Check sheet for the modelled part. Datum: model origin and axes. Units: mm. A direction names the side the tool comes from. Round coordinates to 2 decimals unless told otherwise and drop trailing zeros. Write each loop counter-clockwise with the first axis right and the second up, starting at its lowest first coordinate (ties: lowest second). Pieces come first, ordered by that corner, then holes.
from build123d import *

# Parameters (mm, degrees)
ESQUISSE2_W                 = 220
ESQUISSE2_H                 = 30
T_LE_DE_BASE_PLI_E1_DEPTH   = 4
PLI_START                   = -15
PLI_ESQUISS_1_DEPTH         = 30
PLI_ESQUISS_1_2_DEPTH       = 30
ESQUISSE9_R                 = 4.5
ESQUISSE9_R_2               = 1.25
BOSS_EXTRU_1_DEPTH          = 1.5
ENL_V_START                 = -4
ENL_V_MAT_EXTRU_1_OUTLINE_R = 1.25
ENL_V_MAT_EXTRU_1_DEPTH     = 4
BOSS_EXTRU_2_DEPTH          = 12
BOSS_EXTRU_2_DEPTH_BACK     = 58
ESQUISSE11_W                = 2.5
ESQUISSE11_H                = 30
BOSS_EXTRU_3_DEPTH          = 3
ESQUISSE13_R                = 2
ENL_V_MAT_EXTRU_2_DEPTH     = 1.5
ENL_V_MAT_EXTRU_3_REACH     = 127.256
ESQUISSE14_W                = 1
ESQUISSE14_H                = 17
ESQUISSE12_R                = 1.75
ENL_V_MAT_EXTRU_4_DEPTH     = 223.720608774
ESQUISSE12_7_R              = 5.25
ESQUISSE12_7_R_2            = 1.75
ENL_V_MAT_EXTRU_5_DEPTH     = 223.720608774
BOSS_EXTRU_4_START          = -15
BOSS_EXTRU_4_DEPTH          = 30


# Read off the part's stored shape, not the designer's step: Pli esquissé1, Enlèv. mat.-Extru.1, Boss.-Extru.4
# Sheet-metal steps are written as plain solids
with BuildPart() as part:
    # Esquisse2 → Tôle de base pliée1 (new body)
    with BuildSketch(Plane(origin=(0, 0, 0), x_dir=(1, 0, 0), z_dir=(0, 1, 0))):
        Rectangle(ESQUISSE2_W, ESQUISSE2_H)
    extrude(amount=-T_LE_DE_BASE_PLI_E1_DEPTH)

    # Pli esquissé1 outline → Pli esquissé1 (cut)
    with BuildSketch(Plane.XY.offset(PLI_START)):
        with BuildLine():
            Line((110, 0), (87.480931171, 0))
            Line((87.480931171, 0), (81.651859795, -3.365415928))
            ThreePointArc((81.651859795, -3.365415928), (80.509482084, -3.838604269), (79.283559795, -4))
            Line((79.283559795, -4), (110, -4))
            Line((110, -4), (110, 0))
        make_face()
    extrude(amount=PLI_ESQUISS_1_DEPTH, mode=Mode.SUBTRACT)

    # Pli esquiss_1 2 outline → Pli esquiss_1 2 (add)
    with BuildSketch(Plane.XY.offset(PLI_START)):
        with BuildLine():
            Line((87.480931171, 0), (107.012166491, 11.27636397))
            Line((107.012166491, 11.27636397), (105.012166491, 14.740465585))
            Line((105.012166491, 14.740465585), (79.651859795, 0.098685688))
            ThreePointArc((79.651859795, 0.098685688), (79.474205904, 0.025099036), (79.283559795, 0))
            Line((79.283559795, 0), (87.480931171, 0))
        make_face()
    extrude(amount=PLI_ESQUISS_1_2_DEPTH)

    # Esquisse9 → Boss.-Extru.1 (add)
    # profile 1 of 4: a face of its own
    with BuildSketch(Plane(origin=(19.870232793, -34.416252755, 0), x_dir=(0.8660254037844382, 0.5000000000000011, 0), z_dir=(-0.5000000000000011, 0.8660254037844382, 0))):
        with Locations(Location((80.313436681, 10.5, 0), (0, 0, 90))):
            Circle(ESQUISSE9_R)
        with Locations(Location((80.313436681, 10.5, 0), (0, 0, 180))):
            Circle(ESQUISSE9_R_2, mode=Mode.SUBTRACT)
    # profile 2 of 4: a face of its own
    with BuildSketch(Plane(origin=(19.870232793, -34.416252755, 0), x_dir=(0.8660254037844382, 0.5000000000000011, 0), z_dir=(-0.5000000000000011, 0.8660254037844382, 0))):
        with Locations((93.813436681, 10.5)):
            Circle(ESQUISSE9_R)
        with Locations(Location((93.813436681, 10.5, 0), (0, 0, 180))):
            Circle(ESQUISSE9_R_2, mode=Mode.SUBTRACT)
    # profile 3 of 4: a face of its own
    with BuildSketch(Plane(origin=(19.870232793, -34.416252755, 0), x_dir=(0.8660254037844382, 0.5000000000000011, 0), z_dir=(-0.5000000000000011, 0.8660254037844382, 0))):
        with Locations((93.813436681, -10.5)):
            Circle(ESQUISSE9_R)
        with Locations((93.813436681, -10.5)):
            Circle(ESQUISSE9_R_2, mode=Mode.SUBTRACT)
    # profile 4 of 4: a face of its own
    with BuildSketch(Plane(origin=(19.870232793, -34.416252755, 0), x_dir=(0.8660254037844382, 0.5000000000000011, 0), z_dir=(-0.5000000000000011, 0.8660254037844382, 0))):
        with Locations((80.313436681, -10.5)):
            Circle(ESQUISSE9_R)
        with Locations((80.313436681, -10.5)):
            Circle(ESQUISSE9_R_2, mode=Mode.SUBTRACT)
    extrude(amount=BOSS_EXTRU_1_DEPTH)

    # Enlèv. mat.-Extru.1 outline → Enlèv. mat.-Extru.1 (cut)
    with BuildSketch(Plane(origin=(19.870232793, -34.416252755, 0), x_dir=(0.8660254037844382, 0.5000000000000011, 0), z_dir=(-0.5000000000000011, 0.8660254037844382, 0)).offset(ENL_V_START)):
        with Locations((93.813436681, 10.5)):
            Circle(ENL_V_MAT_EXTRU_1_OUTLINE_R)
        with Locations((93.813436681, -10.5)):
            Circle(ENL_V_MAT_EXTRU_1_OUTLINE_R)
        with Locations((80.313436681, 10.5)):
            Circle(ENL_V_MAT_EXTRU_1_OUTLINE_R)
        with Locations((80.313436681, -10.5)):
            Circle(ENL_V_MAT_EXTRU_1_OUTLINE_R)
    extrude(amount=ENL_V_MAT_EXTRU_1_DEPTH, mode=Mode.SUBTRACT)

    # Esquisse11 → Boss.-Extru.2 (add, two sides: drawn at the far end of the back side and taken through both)
    with BuildSketch(Plane(origin=(0, 0, 0), x_dir=(1, 0, 0), z_dir=(0, 1, 0)).offset(-BOSS_EXTRU_2_DEPTH_BACK)):
        with Locations((-108.75, 0)):
            Rectangle(ESQUISSE11_W, ESQUISSE11_H)
    extrude(amount=BOSS_EXTRU_2_DEPTH + BOSS_EXTRU_2_DEPTH_BACK)

    # Esquisse3D1 → Boss.-Extru.3 (add, along a direction that is not the sketch's normal)
    with BuildSketch(Plane(origin=(-107.5, -58, -15), x_dir=(0.43685202833051884, 0.7863336509949341, 0.43685202833051917), z_dir=(0.8741572761215378, -0.4856429311786321, 0))):
        Polygon((0, 0), (13.10556085, 26.98600146), (68.673138854, 0), (55.567578004, -26.98600146), align=None)
    extrude(amount=-BOSS_EXTRU_3_DEPTH, dir=(0, -1, 0))

    # Esquisse13 → Enlèv. mat.-Extru.2 (cut)
    with BuildSketch(Plane(origin=(21.870232793, -37.88035437, 0), x_dir=(0.8660254037844382, 0.500000000000001, 0), z_dir=(0.500000000000001, -0.8660254037844382, 0))):
        with Locations((93.813436681, 10.5)):
            Circle(ESQUISSE13_R)
        with Locations((93.813436681, -10.5)):
            Circle(ESQUISSE13_R)
        with Locations((80.313436681, -10.5)):
            Circle(ESQUISSE13_R)
        with Locations((80.313436681, 10.5)):
            Circle(ESQUISSE13_R)
    extrude(amount=-ENL_V_MAT_EXTRU_2_DEPTH, mode=Mode.SUBTRACT)

    # Esquisse14 → Enlèv. mat.-Extru.3 (cut, up to next)
    with BuildSketch(Plane(origin=(0, 0, 0), x_dir=(1, 0, 0), z_dir=(0, 1, 0)), mode=Mode.PRIVATE) as enl_v_mat_extru_3_sk1:
        with Locations((67.783559795, 0)):
            Rectangle(ESQUISSE14_W, ESQUISSE14_H)
    enl_v_mat_extru_3_tool1 = extrude(enl_v_mat_extru_3_sk1.sketch, amount=-ENL_V_MAT_EXTRU_3_REACH, mode=Mode.PRIVATE) & part.part
    add(enl_v_mat_extru_3_tool1.solids().sort_by_distance((67.78356, 0, 0))[0], mode=Mode.SUBTRACT)

    # Esquisse12 → Enlèv. mat.-Extru.4 (cut, through all)
    with BuildSketch(Plane(origin=(-107.5, 0, 0), x_dir=(0, 0, -1), z_dir=(1, 0, 0))):
        with Locations((0, -33)):
            Circle(ESQUISSE12_R)
        with Locations((-6.598263909, 8)):
            Circle(ESQUISSE12_R)
        with Locations((7.051423878, 8)):
            Circle(ESQUISSE12_R)
    extrude(amount=-ENL_V_MAT_EXTRU_4_DEPTH, mode=Mode.SUBTRACT)

    # Esquisse12<7> → Enlèv. mat.-Extru.5 (cut, through all)
    # profile 1 of 2: a face of its own
    with BuildSketch(Plane(origin=(-107.5, 0, 0), x_dir=(0, 0, -1), z_dir=(1, 0, 0))):
        with Locations(Location((0, -33, 0), (0, 0, 270))):
            Circle(ESQUISSE12_7_R)
        with Locations((0, -33)):
            Circle(ESQUISSE12_7_R_2, mode=Mode.SUBTRACT)
    # profile 2 of 2: a face of its own
    with BuildSketch(Plane(origin=(-107.5, 0, 0), x_dir=(0, 0, -1), z_dir=(1, 0, 0))):
        with Locations(Location((0, -33, 0), (0, 0, 270))):
            Circle(ESQUISSE12_7_R)
    extrude(amount=ENL_V_MAT_EXTRU_5_DEPTH, mode=Mode.SUBTRACT)

    # Boss.-Extru.4 outline → Boss.-Extru.4 (add)
    with BuildSketch(Plane.XY.offset(BOSS_EXTRU_4_START)):
        Polygon((-107.5, -4), (-107.5, -8), (-103.5, -4), align=None)
        Polygon((-103.5, 0), (-107.5, 4), (-107.5, 0), align=None)
    extrude(amount=BOSS_EXTRU_4_DEPTH)


solid = part.part
1. Sectioned sample at A-A, the plane y = -51. Enter the section's corners in (x, z), plus the area to 3 significant figures.
2. Set-up check for faces 1 (the cylindrical face through (102.41, 12.63, 10.12)), 2 (the flat face through (-105.5, -6, -0.2)), 3 (the flat face through (104.23, 14.29, 13.91)), 4 (the flat face through (67.284, -2, 0)), 5 (the flat face through (-13, 0, 0)): record each of +Z, -Z, +X, -X, +Y, -Y from which the full face is reachable in a straight line by a thin tool's end or side.
3. Scan lines: line 1 along Y through (x, z) = (-108.6, 0); line 2 along Y through (x, z) = (43.5, 12); line 3 along Z through (x, y) = (-94, -33). Record each from-to range of solid material in increasing order.
4. Sectioned sample at B-B, the plane x = -35.5. Enter the section's corners in (y, z), plus the area to 3 significant figures.
5. Go/stop test with flat-tipped pins: pin 1 (2 mm diameter, centred on x = -109, z = 6, fed in from +Y); pin 2 (3 mm diameter, centred on y = 8, z = 6.6, fed in from +X); pin 3 (5 mm diameter, centred on y = -38, z = -8, fed in from +X). Record where each tip stops, or that it passes through.
Computed values:
1. outline: (-110, -15) - (-107.5, -15) - (-107.5, 15) - (-110, 15) - close; (-105.28, -15) - (-103.61, -15) - (-103.61, 15) - (-105.28, 15) - close
1. area: 125 mm2
2. face 1: none
2. face 2: +Z, -Z
2. face 3: +Z, +Y
2. face 4: +Y, -Y
2. face 5: +Z, -Z, +Y
3. line 1: y = -58 to -34.75, -31.25 to 12
3. line 2: y = -4 to 0
3. line 3: z = -15 to -5.25, 5.25 to 15
4. outline: (-4, -15) - (0, -15) - (0, 15) - (-4, 15) - close
4. area: 120 mm2
5. pin 1: stops at y = 12
5. pin 2: stops at x = 103.94
5. pin 3: stops at x = -95
